Build history of the part. All positions in model axes, mm. A direction names the side the tool comes from. Round coordinates to 2 decimals unless told otherwise and drop trailing zeros. Write each loop counter-clockwise with the first axis right and the second up, starting at its lowest first coordinate (ties: lowest second). Pieces come first, ordered by that corner, then holes.
Item 1: Drop flat-ended pins along their axis: pin 1 Ø2.5 at (x, y) = (3, 90) entering from +Z; pin 2 Ø5 at (x, z) = (-1.5, -2) entering from +Y; pin 3 Ø1.5 at (x, y) = (0.5, 92.5) entering from -Z; pin 4 Ø5 at (x, y) = (-3.5, 35) entering from -Z. Give the stop position or say it passes through.
Item 2: 3-axis set-ups, long thin cutter, end or side, ignore diameter. For faces 4 (the cylindrical face through (2, 112, 0)), 5 (the cylindrical face through (0.57, 65.81, 4.9)), 6 (the cylindrical face through (0.6, 65.81, -4.93)), 7 (the flat face through (0, 64, 0)), 8 (the flat face through (4, 64, -5.5)): which of +Z, -Z, +X, -X, +Y, -Y reach the whole face in a straight line?
Item 3: Band-saw the part on B-B, the plane y = 115. Write the cut outline in (x, z).
Item 4: Band-saw the part on A-A, the plane z = 0. Write the cut outline in (x, y), then the cut area to 3 significant figures.
Item 5: Band-saw the part on C-C, the plane y = 87.5. Write the cut outline in (x, z).
Item 6: Wall check: probe 1 along Y at (x, z) = (2.4, 0); probe 2 along Y at (x, z) = (1, 0); probe 3 along Z at (x, y) = (3.1, 115). Give the ranges that are in metal, low to high.
Item 7: Mould opens along Z. For faces 1 (the cylindrical face through (2, 32, 0)), 2 (the flat face through (3, 64, 5.5)), 3 (the flat face through (-2.2, 5, 0.1)) say: +Z half, -Z half, draft (parallel to the pull), parting line (faces both ways), or undercut.
Autodesk Inventor part; units mm, degrees
ref_plane "YZ Plane" through (0, 0, 0) normal (1, 0, 0) x (0, 1, 0)
ref_plane "XZ Plane" through (0, 0, 0) normal (0, 1, 0) x (-1, 0, 0)
ref_plane "XY Plane" through (0, 0, 0) normal (0, 0, 1) x (1, 0, 0)
sketch "スケッチ1" plane through (0, 0, 0) normal (0, 1, 0) x (-1, 0, 0)
  line L0 (5, -10) -> (-5, -10)
  line L1 (-5, -10) -> (-5, 10)
  line L2 (-5, 10) -> (5, 10)
  line L3 (5, 10) -> (5, -10)
  line L4 (5, -10) -> (-5, 10) construction
  line L5 (-5, -10) -> (5, 10) construction
  point P0 (0, 0)
  dimension "d0" = 10
  dimension "d1" = 20
extrude "押し出し1" add sketch "スケッチ1" along normal blind 5
sketch "スケッチ4" plane through (0, 5, 0) normal (0, 1, 0) x (1, 0, 0)
  line L0 (5, 5.5) -> (0, 5.5)
  line L1 (0, 5.5) -> (0, -5.5)
  line L2 (0, -5.5) -> (5, -5.5)
  line L3 (5, -5.5) -> (5, 5.5)
  line L4 (5, -10) -> (5, 10)
  point P0 (0, 0)
  dimension "d11" = 5
  dimension "d12" = 11
  dimension "d13" = 5
  dimension "d14" = 5.5
extrude "押し出し4" add sketch "スケッチ4" along normal blind 120
sketch "スケッチ6" plane through (5, 0, 10) normal (1, 0, 0) x (0, 0, -1)
  line L0 (4.5, 5) -> (15.5, 5)
  line L1 (15.5, 5) -> (15.5, 125)
  point P0 (10, 0)
  point P1 (10, 35)
  point P2 (10, 115)
  dimension "d30" = 30
  dimension "d31" = 80
  dimension "d32" = 5.5
  dimension "d33" = 5.5
hole "穴2" at (5, 35, 0) at (5, 115, 0) direction (-1, 0, 0) diameter 6 end through all
fillet "フィレット3" radius 2 8 edges at (2.5, 125, 5.5) (2.5, 125, -5.5) (0, 125, 0) (0, 65, 5.5) (0, 65, -5.5) (2.5, 5, 5.5) (0, 5, 0) (2.5, 5, -5.5)
properties part number "baseB"
Results:
1. pin 1: stops at z = 5.5
1. pin 2: stops at y = 124.73
1. pin 3: stops at z = -5.35
1. pin 4: passes through
2. face 4: +X, -X
2. face 5: +Z, -X, +Y
2. face 6: -Z, -X, +Y
2. face 7: +Z, -Z, -X, +Y
2. face 8: -Z, +X, -X, +Y
3. outline: (0, -3.5) arc R2 ccw to (2, -5.5) - (5, -5.5) - (5, -3) - (0, -3) - close; (0, 3) - (5, 3) - (5, 5.5) - (2, 5.5) arc R2 ccw to (0, 3.5) - close
4. outline: (-5, 0) - (5, 0) - (5, 32) - (0, 32) - (0, 7) arc R2 cw to (-2, 5) - (-5, 5) - close; (0, 38) - (5, 38) - (5, 112) - (0, 112) - close; (0, 118) - (5, 118) - (5, 125) - (2, 125) arc R2 ccw to (0, 123) - close
4. area: 590 mm2
5. outline: (0, -3.5) arc R2 ccw to (2, -5.5) - (5, -5.5) - (5, 5.5) - (2, 5.5) arc R2 ccw to (0, 3.5) - close
6. probe 1: y = 0 to 32, 38 to 112, 118 to 125
6. probe 2: y = 0 to 32, 38 to 112, 118 to 124.73
6. probe 3: z = -5.5 to -3, 3 to 5.5
7. face 1: undercut
7. face 2: +Z half
7. face 3: draft
